Autodesk Inventor part; units mm, degrees
ref_plane "Work Plane1" through (-41.89, 79.898, 0.7952) normal (0, 0, 1) x (1, 0, 0)
ref_plane "YZ Plane" through (0, 0, 0) normal (1, 0, 0) x (0, 1, 0)
ref_plane "XZ Plane" through (0, 0, 0) normal (0, 1, 0) x (-1, 0, 0)
ref_plane "Work Plane1" through (-41.89, 79.898, 0.7952) normal (0, 0, 1) x (1, 0, 0)
sketch "Sketch1" plane through (-41.89, 79.898, 0.7952) normal (0, 0, 1) x (1, 0, 0)
  circle A0 centre (41.89, -79.898) radius 1.45
  circle A1 centre (8.87, -27.828) radius 1.45
  circle A2 centre (57.13, -29.098) radius 1.45
  arc A3 (66, -80.398) -> (68, -78.398) centre (66, -78.398) ccw
  line L0 (66, 0.102) -> (0, 0.102)
  line L1 (-2, -1.898) -> (-2, -24.398)
  line L2 (-2, 0.102) -> (68, 0.102)
  line L3 (68, 0.102) -> (68, -82.398)
  line L4 (68, -82.398) -> (-2, -82.398)
  line L5 (-2, -82.398) -> (-2, 0.102)
  line L6 (-2, 3.102) -> (-5, 3.102)
  line L7 (68, -85.398) -> (71, -85.398)
  line L8 (-5, 3.102) -> (71, 3.102)
  line L9 (71, 3.102) -> (71, -85.398)
  line L10 (71, -85.398) -> (-5, -85.398)
  line L11 (-5, -85.398) -> (-5, 3.102)
  point P0 (44.5, -82.398)
  point P1 (-2, 3.102)
  point P2 (-2, -24.398)
  point P3 (-2, -1.898)
  point P4 (66, 0.102)
  dimension "d0" = 2.9
  dimension "d1" = 2.9
  dimension "d2" = 2.9
extrude "Extrusion1" add sketch "Sketch1" against normal blind 3 contours L2 L3 L4 L5 L1 L0 | L8 L9 L7 L10 L11 L6
sketch "Sketch2" plane through (-41.89, 79.898, 0.7952) normal (0, 0, 1) x (1, 0, 0)
  circle A0 centre (8.87, -27.828) radius 1.45
  circle A1 centre (8.87, -27.828) radius 3
  circle A2 centre (57.13, -29.098) radius 1.45
  circle A3 centre (57.13, -29.098) radius 3
  circle A4 centre (41.89, -79.898) radius 3
  circle A5 centre (41.89, -79.898) radius 1.45
  dimension "d9" = 6
  dimension "d10" = 6
  dimension "d11" = 6
extrude "Extrusion2" add sketch "Sketch2" along normal blind 3
sketch "Sketch3" plane through (-41.89, 79.898, 0.7952) normal (0, 0, 1) x (1, 0, 0)
  line L0 (71, -85.398) -> (-5, -85.398)
  circle A0 centre (18, -27.898) radius 1.45
  circle A1 centre (48, -27.898) radius 1.45
  circle A2 centre (18, -57.898) radius 1.45
  circle A3 centre (48, -57.898) radius 1.45
  point P0 (41.89, -79.898)
  dimension "d19" = 2.9
  dimension "d20" = 2.9
  dimension "d21" = 2.9
  dimension "d22" = 2.9
extrude "Extrusion3" cut sketch "Sketch3" against normal up to surface (3 mm away)
extrude "Extrusion5" add sketch "Sketch1" along normal blind 4.58 contours L8 L9 L7 L10 L11 L6
sketch "Sketch5" plane through (-41.89, 79.898, 5.3752) normal (0, 0, 1) x (1, 0, 0)
  line L0 (-2, 0.102) -> (-2, -82.398)
  line L1 (-2, -82.898) -> (68, -82.898)
  line L2 (43.5483, -82.398) -> (68, -82.398)
  line L3 (68, -82.898) -> (68.5, -82.898)
  line L4 (68.5, -82.898) -> (68.5, 0.102)
  line L5 (68, -82.398) -> (68, 0.102)
  line L6 (68.5, 0.102) -> (68.5, 0.602)
  line L7 (68.5, 0.602) -> (-2, 0.602)
  line L8 (-2, 0.602) -> (-2.5, 0.602)
  line L9 (-2.5, 0.602) -> (-2.5, -82.898)
  line L10 (-2.5, -82.898) -> (-2, -82.898)
  line L11 (-2, -82.398) -> (-2, 0.102)
  line L12 (68, -82.398) -> (-2, -82.398)
  line L13 (68, 0.102) -> (68, -82.398)
  line L14 (-2, 0.102) -> (68, 0.102)
  point P0 (41.89, -79.898)
  dimension "d33" = 0.5
  dimension "d34" = 0.5
  dimension "d35" = 0.5
  dimension "d36" = 0.5
extrude "Extrusion6" cut sketch "Sketch5" against normal up to surface (4.58 mm away)
sketch "Sketch6" plane through (-41.89, 79.898, 0.7952) normal (0, 0, 1) x (1, 0, 0)
  circle A0 centre (48, -57.898) radius 1.45
  circle A1 centre (18, -57.898) radius 1.45
  circle A2 centre (48, -47.966) radius 4.767
  circle A3 centre (18, -47.966) radius 4.767
  point P0 (41.89, -79.898)
  dimension "d40" = 9.534
extrude "Extrusion7" cut sketch "Sketch6" against normal up to surface (3 mm away) contours A2 | A3
sketch "Sketch7" plane through (15.24, 50.8, 3.7952) normal (0, 0, 1) x (1, 0, 0)
  line L0 (-16.8983, -53.3) -> (-13.5817, -53.3)
  arc A0 (-13.5817, -53.3) -> (-16.8983, -53.3) centre (-15.24, -50.8) ccw
  circle A1 centre (-15.24, -50.8) radius 1.45
  circle A2 centre (-48.26, 1.27) radius 3
  circle A3 centre (-48.26, 1.27) radius 1.45
  circle A4 centre (0, 0) radius 3
  circle A5 centre (0, 0) radius 1.45
  point P0 (-15.24, -50.8)
extrude "Extrusion8" add sketch "Sketch7" along normal blind 5
sketch "Sketch8" plane through (-41.89, 79.898, 5.3752) normal (0, 0, 1) x (1, 0, 0)
  line L0 (68.5, -82.898) -> (-2.5, -82.898)
  line L1 (-2.5, -82.898) -> (-2.5, 0.602)
  line L2 (-2.5, 0.602) -> (68.5, 0.602)
  line L3 (68.5, 0.602) -> (68.5, -82.898)
  line L4 (71, 3.102) -> (-5, 3.102)
  line L5 (-5, 3.102) -> (-5, -85.398)
  line L6 (-5, -85.398) -> (71, -85.398)
  line L7 (71, -85.398) -> (71, 3.102)
  point P0 (41.89, -79.898)
extrude "Extrusion9" add sketch "Sketch8" along normal blind 5
sketch "Sketch9" plane through (15.24, 50.8, 8.7952) normal (0, 0, 1) x (1, 0, 0)
  circle A0 centre (0, 0) radius 1.45
  circle A1 centre (0, 0) radius 3
  line L0 (0, 0) -> (0, -2)
  line L1 (0, -2) -> (2.2361, -2)
  line L2 (0, -2) -> (-2.2361, -2)
  point P0 (-15.24, -50.8)
  dimension "d47" = 2
extrude "Extrusion10" cut sketch "Sketch9" against normal up to surface (8 mm away) contours L1 A1 L2 picked at (1.3106, -2.1582)
sketch "Sketch10" plane through (-41.89, 79.898, 0.7952) normal (0, 0, 1) x (1, 0, 0)
  arc A0 (43.5483, -82.398) -> (40.2317, -82.398) centre (41.89, -79.898) ccw
  circle A1 centre (41.89, -79.898) radius 3
  circle A2 centre (41.89, -79.898) radius 1.45
  circle A3 centre (41.89, -79.898) radius 1.45
  point P0 (41.89, -79.898)
  point P1 (40.2317, -82.398)
extrude "Extrusion11" add sketch "Sketch10" along normal up to surface (8 mm away)
properties part number "nucleo_din_connector"
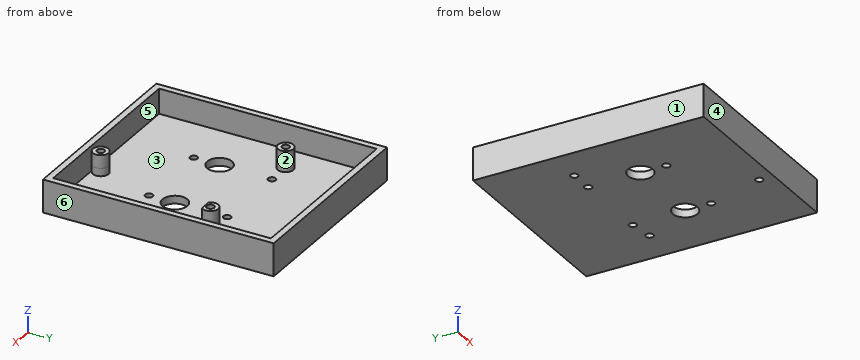
Check sheet for the modelled part. Datum: model origin and axes. Units: mm. Face numbers are marked on the shaded views. A direction names the side the tool comes from. Give positions to 0.01 mm unless a question says otherwise; leave off trailing zeros. Order: outer loops, then holes, each group sorted by start corner. A loop starts at its lowest first (then second) coordinate and runs counter-clockwise, first axis right, second up. Notation, with made-up numbers: (85, 78.25) -> (131, 78.25) arc R18 ccw to (131, 99.25) -> close; hole circle Ø4 at (68, 15.5). An arc over 180 degrees is marked (long way). Use CSV: the item, a comma, the result in double quotes. Start each with the question number.
1) Sectioned sample at D-D, the plane y = 64. Record the boundary of the cut face in (x, z), plus the area to 3 significant figures.
2) Material ranges on line 1 (Y direction, x = 6.11, z = -0.4) (3 decimals); line 2 (Y direction, x = -33.02, z = 3.5); line 3 (X direction, y = 71, z = 9.25), recorded low to high. Write a range as from..to.
3) Mould release check, pull along Y, two halves, no side actions. Record for the marked faces 3, 4, 5 and 6: released by +Y, released by -Y, zero draft, split by the parting line, or undercut.
4) Set-up check for the marked faces 1 and 2: record each of +Z, -Z, +X, -X, +Y, -Y from which the full face is reachable in a straight line by a thin tool's end or side.
5) Go/stop test with flat-tipped pins: P1, Ø10, axis at x = -18.5, y = 60, coming from the +Z side; P2, Ø3.5, axis at x = -33.02, y = 52.07, coming from the -Z side; P3, Ø3, axis at x = -32, y = 52.5, coming from the +Z side. Record where each tip stops, or that it passes through.
6) Sectioned sample at C-C, the plane z = 7. Record the boundary of the cut face in (x, y), plus the area to 3 significant figures.
7) Sectioned sample at B-B, the plane x = 6.11. Record the boundary of the cut face in (y, z) (3 decimals), plus the area to 3 significant figures.
8) Sectioned sample at A-A, the plane y = 0. Record the boundary of the cut face in (x, z).
Recorded:
1,outline,"(-46.89, -2.2) -> (29.11, -2.2) -> (29.11, 10.38) -> (26.61, 10.38) -> (26.61, 0.8) -> (-44.39, 0.8) -> (-44.39, 10.38) -> (-46.89, 10.38) -> close"
1,area,"276 mm2"
2,line 1,"-5.5..20.55, 23.45..27.165, 36.699..50.55, 53.45..83"
2,line 2,"-5.5..-3, 49.07..50.62, 53.52..55.07, 80.5..83"
2,line 3,"-46.89..-44.39, 26.61..29.11"
3,face 3,"undercut"
3,face 4,"released by -Y"
3,face 5,"undercut"
3,face 6,"zero draft"
4,face 1,"+Z, -Z, -X, +Y, -Y"
4,face 2,"+Z"
5,P1,"z = 0.8"
5,P2,"z = -2.2"
5,P3,"z = 8.8"
6,outline,"(-46.89, -5.5) -> (29.11, -5.5) -> (29.11, 83) -> (-46.89, 83) -> close; circle Ø6 at (-33.02, 52.07); (0, -3) arc R3 ccw to (1.66, -2.5) arc R3 ccw (long way) to start; (13, 48.8) -> (17.48, 48.8) arc R3 ccw (long way) to start; hole (-44.39, -3) -> (26.61, -3) -> (26.61, 80.5) -> (-44.39, 80.5) -> close; hole circle Ø2.9 at (-33.02, 52.07); hole circle Ø2.9 at (0, 0); hole circle Ø2.9 at (15.24, 50.8)"
6,area,"859 mm2"
7,outline,"(-5.5, -2.205) -> (20.55, -2.205) -> (20.55, 0.795) -> (-3, 0.795) -> (-3, 10.375) -> (-5.5, 10.375) -> close; (23.45, -2.205) -> (27.165, -2.205) -> (27.165, 0.795) -> (23.45, 0.795) -> close; (36.699, -2.205) -> (50.55, -2.205) -> (50.55, 0.795) -> (36.699, 0.795) -> close; (53.45, -2.205) -> (83, -2.205) -> (83, 10.375) -> (80.5, 10.375) -> (80.5, 0.795) -> (53.45, 0.795) -> close"
7,area,"267 mm2"
8,outline,"(-46.89, -2.2) -> (-1.45, -2.2) -> (-1.45, 8.8) -> (-3, 8.8) -> (-3, 0.8) -> (-44.39, 0.8) -> (-44.39, 10.38) -> (-46.89, 10.38) -> close; (1.45, -2.2) -> (29.11, -2.2) -> (29.11, 10.38) -> (26.61, 10.38) -> (26.61, 0.8) -> (3, 0.8) -> (3, 8.8) -> (1.45, 8.8) -> close"
